Here's how the part is built. I have some questions about the finished solid (model axes, mm). A direction names the side the tool comes from. Round coordinates to 2 decimals unless told otherwise and drop trailing zeros. Write each loop counter-clockwise with the first axis right and the second up, starting at its lowest first coordinate (ties: lowest second). Pieces come first, ordered by that corner, then holes. Notation, with made-up numbers: (-3, -26.75) - (46, -26.75) arc R24 cw to (46, -5.75) - close; hole circle Ø9 at (87.5, 6.5). An arc over 180 degrees is marked (long way). One line per item, written item: value. Start each with the question number.
Item 1: Imagine slicing it at D-D, the plane x = 6.75. Please give me the cut outline in (y, z).
Item 2: Thinking about a two-plate mould opening in X: for faces 3 (the face through (4, 2.871, 21)), 4 (the face through (13.076, 4.054, 22.217)), 5 (the face through (13.913, 4.89, 33.374)), 6 (the face through (4, 1, 46)), which applies, released by +X, released by -X, zero draft, split by the parting line, or undercut?
Item 3: For faces 1 (the face through (8, 2, 27)), 2 (the face through (12.95, 3.93, 40.95)), which set-ups out of +Z, -Z, +X, -X, +Y, -Y let a thin tool reach every point of the face, with its end or its side?
Item 4: Imagine slicing it at C-C, the plane z = 51. Please give me the cut outline in (x, y).
Item 5: For P1, Ø9, axis at x = 4.5, z = 37.5, coming from the +Y side; P2, Ø4, axis at y = 1.5, z = 49, coming from the -X side; P3, Ø2, axis at x = 2, y = 1.5, coming from the -Z side, each with a flat end and sliding along its axis, tell me the tip position at first contact or that it passes through.
Item 6: Imagine slicing it at A-A, the plane y = 2. Please give me the cut outline in (x, z), then the cut area to 3 significant figures.
Item 7: Imagine slicing it at B-B, the plane z = 20. Please give me the cut outline in (x, y).
Item 8: If I drill on line 1 (Y direction, x = 10.25, z = 16); line 2 (X direction, y = 0.75, z = 3); line 3 (Y direction, x = 4, z = 39), over which ranges is the centre line in solid material (lowest first)?
```python
from build123d import *

# Parameters (mm, degrees)
EXTRUDE_1_DEPTH        = 63.5
SKETCH_2_R             = 1.45
EXTRUDE_2_DEPTH        = 2.5
SKETCH_3_R             = 2
EXTRUDE_3_DEPTH        = 0.5
PATTERN_LINEAR_1_COUNT = 9
PATTERN_LINEAR_1_PITCH = 7.4
SKETCH_4_R             = 1.6
CUT_EXTRUDE_1_DEPTH    = 10.5
PATTERN_LINEAR_2_COUNT = 3
PATTERN_LINEAR_2_PITCH = 15
CUT_EXTRUDE_2_DEPTH    = 5
FILLET_1_R             = 6
FILLET_2_R             = 4


with BuildPart() as part:
    # 草图1 → 凸台-拉伸1 (new body)
    with BuildSketch(Plane.XY):
        Polygon((16.9, 0), (16.9, 3.426641456), (14.8489809, 5.477660556), (14.495427509, 5.124107166), (12.374107166, 3.002786822), (10.871320344, 1.5), (8, 1.5), (8, 2.871320344), (0, 2.871320344), (0, 0), align=None)
    extrude(amount=EXTRUDE_1_DEPTH)

    # 草图2 → 凸台-拉伸2 (add)
    with BuildSketch(Plane(origin=(4.685660172, -4.685660172, 0), x_dir=(0, 0, 1), z_dir=(-0.7071067811865562, 0.7071067811865389, 0))):
        with Locations(Location((2, 12.373106012, 0), (0, 0, 90))):
            Circle(SKETCH_2_R)
    extrude_2 = extrude(amount=EXTRUDE_2_DEPTH)

    # 草图3 → 凸台-拉伸3 (add)
    with BuildSketch(Plane(origin=(4.685660172, -4.685660172, 0), x_dir=(0, 0, 1), z_dir=(-0.7071067811865562, 0.7071067811865389, 0))):
        with Locations(Location((2, 12.373106012, 0), (0, 0, 90))):
            Circle(SKETCH_3_R)
    extrude_3 = extrude(amount=EXTRUDE_3_DEPTH)

    # 阵列(线性)1: 凸台-拉伸2, 凸台-拉伸3 ×9
    with Locations(*[(0, 0, i * PATTERN_LINEAR_1_PITCH) for i in range(1, PATTERN_LINEAR_1_COUNT)]):
        add(extrude_2)
        add(extrude_3)

    # 草图4 → 切除-拉伸1 (cut)
    with BuildSketch(Plane(origin=(0, 2.871320344, 0), x_dir=(1, 0, 0), z_dir=(0, 1, 0))):
        with Locations(Location((4, -4, 0), (0, 0, 180))):
            Circle(SKETCH_4_R)
    cut_extrude_1 = extrude(amount=-CUT_EXTRUDE_1_DEPTH, mode=Mode.SUBTRACT)

    # 阵列(线性)2: 切除-拉伸1 ×3
    with Locations(*[(0, 0, i * PATTERN_LINEAR_2_PITCH) for i in range(1, PATTERN_LINEAR_2_COUNT)]):
        add(cut_extrude_1, mode=Mode.SUBTRACT)

    # 草图6 → 切除-拉伸2 (cut, symmetric)
    with BuildSketch(Plane(origin=(0, 2.871320344, 0), x_dir=(1, 0, 0), z_dir=(0, 1, 0))):
        with BuildLine():
            Line((4, -40.973787182), (0.723391823, -36.294305745))
            ThreePointArc((0.723391823, -36.294305745), (0.185132197, -35.202823198), (0, -34))
            Line((0, -34), (-4.848158237, -34))
            Line((-4.848158237, -34), (-4.848158237, -69.568318456))
            Line((-4.848158237, -69.568318456), (19.447072331, -69.568318456))
            Line((19.447072331, -69.568318456), (19.447072331, -55.8))
            Line((19.447072331, -55.8), (4, -55.8))
            Line((4, -55.8), (4, -40.973787182))
        make_face()
    extrude(amount=CUT_EXTRUDE_2_DEPTH, both=True, mode=Mode.SUBTRACT)

    # 圆角1
    fillet_1_edges = [part.edges().sort_by_distance(p)[0] for p in [
        (4, 1.435660172, 55.8),
    ]]
    fillet(fillet_1_edges, radius=FILLET_1_R)

    # 圆角2
    fillet_2_edges = [part.edges().sort_by_distance(p)[0] for p in [
        (4, 1.435660172, 40.973787182),
    ]]
    fillet(fillet_2_edges, radius=FILLET_2_R)


solid = part.part
```
Values follow:
1. outline: (0, 0) - (2.87, 0) - (2.87, 54.84) - (0, 54.84) - close
2. face 3: zero draft
2. face 4: undercut
2. face 5: undercut
2. face 6: released by -X
3. face 1: +Z, -Z, +Y
3. face 2: none
4. outline: (4.12, 0) - (16.9, 0) - (16.9, 3.43) - (14.85, 5.48) - (10.87, 1.5) - (8, 1.5) - (8, 2.87) - (4.12, 2.87) - close
5. P1: stops at y = 2.87
5. P2: stops at x = 4
5. P3: stops at z = 0
6. outline: (0, 0) - (8, 0) - (8, 55.46) arc R6 ccw to (4, 49.8) - (4, 42.23) arc R4 cw to (3.28, 39.94) - (0.72, 36.29) arc R4 ccw to (0, 34) - close; (11.37, 0) - (16.9, 0) - (16.9, 55.8) - (11.37, 55.8) - close; hole circle Ø3.2 at (4, 4); hole circle Ø3.2 at (4, 19); hole circle Ø3.2 at (4, 34)
6. area: 653 mm^2
7. outline: (0, 0) - (2.75, 0) - (2.75, 2.87) - (0, 2.87) - close; (5.25, 0) - (16.9, 0) - (16.9, 3.43) - (14.85, 5.48) - (10.87, 1.5) - (8, 1.5) - (8, 2.87) - (5.25, 2.87) - close
8. line 1: y = 0 to 1.5
8. line 2: x = 0 to 2.75, 5.25 to 16.9
8. line 3: y = 0 to 2.87
